from build123d import *

# Parameters (mm, degrees)
SKETCH1_R                 = 12.7
BOSS_EXTRUDE1_DEPTH       = 4.365625
F_6_32_TAPPED_HOLE1_D     = 2.7051
F_6_32_TAPPED_HOLE1_DEPTH = 23.876
F_6_32_TAPPED_HOLE1_TIP   = 0.81269403


with BuildPart() as part:
    # Sketch1 → Boss-Extrude1 (new body)
    with BuildSketch(Plane(origin=(0, 0, 0), x_dir=(1, 0, 0), z_dir=(0, 1, 0))):
        with Locations(Location((0, 0, 0), (0, 0, 270))):
            Circle(SKETCH1_R)
    extrude(amount=BOSS_EXTRUDE1_DEPTH)

    # #6-32 Tapped Hole1
    with Locations(Plane(origin=(0, 4.365625, 0), x_dir=(1, 0, 0), z_dir=(0, 1, 0))):
        with Locations((0, 9.779), (6.914797213, 6.914797213), (9.779, 0), (6.914797213, -6.914797213), (0, -9.779), (-6.914797213, -6.914797213), (-9.779, 0), (-6.914797213, 6.914797213)):
            Hole(F_6_32_TAPPED_HOLE1_D / 2, depth=F_6_32_TAPPED_HOLE1_DEPTH)
            with Locations((0, 0, -(F_6_32_TAPPED_HOLE1_DEPTH + F_6_32_TAPPED_HOLE1_TIP / 2))):  # 118° drill point
                Cone(0, F_6_32_TAPPED_HOLE1_D / 2, F_6_32_TAPPED_HOLE1_TIP, mode=Mode.SUBTRACT)


solid = part.part
The model under review builds one solid part; all positions refer to its coordinate system, in mm. Coordinates: 2 decimals unless noted, no trailing zeros. Loops run counter-clockwise (first coordinate to the right, second up) from the corner with the lowest first, then second, coordinate; pieces in that order, holes last. Notation, with made-up numbers: M 11.5,6 L 21.5,6 A16 cw 21.5,23 Z; hole C 65.25,-11 d7. An arc over 180 degrees is marked long. Put each result on its own line as item: value. Start each with the question number.
Q1. The part is to be moulded in two halves that separate along Z. For faces 1 (the cylindrical face through (0.29, 2.15, 11.1)), 2 (the cylindrical face through (-7.7, 2.2, -10.1)), 3 (the flat face through (0, 4.366, 0)), say which applies: +Z half, -Z half, draft (parallel to the pull), parting line (faces both ways), or undercut.
Q2. Add section C-C (x = 9.5). Write out the cut boundary in (y, z).
Q3. Add section D-D (z = -9.25). Write out the cut boundary in (x, y), and give its area (3 significant figures).
Q4. Add section A-A (z = 0). Write out the cut boundary in (x, y).
Q5. Add section B-B (x = 0). Write out the cut boundary in (y, z).
Q6. Clearance check with flat-ended pins moving along their axes: pin 1 (3 mm diameter, centred on x = 0, z = 9.779, fed in from -Y); pin 2 (1 mm diameter, centred on x = -9.5, y = 3.5, fed in from -Z); pin 3 (2 mm diameter, centred on x = -1.5, y = 2.5, fed in from +Z). State where each tip first meets the part, or that it passes through.
Q7. Wall thickness on line 1 (Z direction, x = -0.25, y = 1.4); line 2 (Z direction, x = 5.75, y = 1.55); line 3 (X direction, y = 1, z = 7.5): over which ranges is each line inside the solid? List them lowest first.
Answers:
1. face 1: undercut
1. face 2: parting line
1. face 3: draft
2. outline: M 0,-8.43 L 4.37,-8.43 L 4.37,-1.32 L 0,-1.32 Z; M 0,1.32 L 4.37,1.32 L 4.37,8.43 L 0,8.43 Z
3. outline: M -8.7,0 L -1.24,0 L -1.24,4.37 L -8.7,4.37 Z; M 1.24,0 L 8.7,0 L 8.7,4.37 L 1.24,4.37 Z
3. area: 65.1 mm^2
4. outline: M -12.7,0 L -11.13,0 L -11.13,4.37 L -12.7,4.37 Z; M -8.43,0 L 8.43,0 L 8.43,4.37 L -8.43,4.37 Z; M 11.13,0 L 12.7,0 L 12.7,4.37 L 11.13,4.37 Z
5. outline: M 0,-12.7 L 4.37,-12.7 L 4.37,-11.13 L 0,-11.13 Z; M 0,-8.43 L 4.37,-8.43 L 4.37,8.43 L 0,8.43 Z; M 0,11.13 L 4.37,11.13 L 4.37,12.7 L 0,12.7 Z
6. pin 1: stops at y = 0
6. pin 2: stops at z = -8.96
6. pin 3: stops at z = 12.69
7. line 1: z = -12.7 to -11.11, -8.45 to 8.45, 11.11 to 12.7
7. line 2: z = -11.32 to -7.6, -6.23 to 6.23, 7.6 to 11.32
7. line 3: x = -10.25 to -8.13, -5.7 to 5.7, 8.13 to 10.25
